Input: part model. Units: mm. Frame: model coordinates. Coordinates: 2 decimals unless noted, no trailing zeros. Loops run counter-clockwise (first coordinate to the right, second up) from the corner with the lowest first, then second, coordinate; pieces in that order, holes last. Notation, with made-up numbers: (-30, -33.5) -> (0, -33.5) arc R14 ccw to (0, -12.5) -> close; hole circle Ø10 at (5.25, 30.5). An arc over 180 degrees is marked (long way). Answer as a JSON object with one key per item and string values.
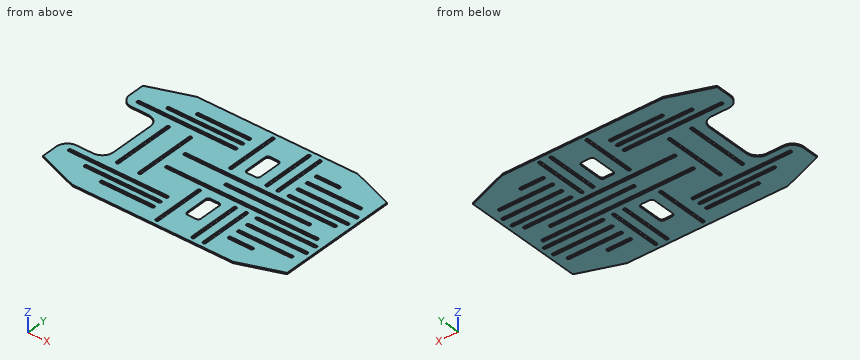
from build123d import *

# Parameters (mm, degrees)
BOSS_EXTRUDE1_DEPTH = 3.175
FILLET3_R           = 25.4
CUT_EXTRUDE3_DEPTH  = 4.175
SCALE1_SCALE        = 0.35


with BuildPart() as part:
    # Sketch1 → Boss-Extrude1 (new body)
    with BuildSketch(Plane.XY):
        Polygon((-279.4, 138.38935405), (-184.214073546, 173.034198), (184.214073546, 173.034198), (279.4, 138.38935405), (279.4, -138.38935405), (184.214073546, -173.034198), (-184.214073546, -173.034198), (-279.4, -138.38935405), (-279.4, -76.2), (-190.5, -76.2), (-190.5, 76.2), (-279.4, 76.2), align=None)
    extrude(amount=BOSS_EXTRUDE1_DEPTH)

    # Fillet3
    fillet3_edges = [part.edges().sort_by_distance(p)[0] for p in [
        (-279.4, -76.2, 1.5875),
        (-190.5, -76.2, 1.5875),
        (-190.5, 76.2, 1.5875),
        (-279.4, 76.2, 1.5875),
    ]]
    fillet(fillet3_edges, radius=FILLET3_R)

    # Sketch4 → Cut-Extrude3 (cut, through all)
    with BuildSketch(Plane.XY.offset(3.175)):
        with BuildLine():
            Line((-254, 98.6282), (-31.75, 98.6282))
            ThreePointArc((-31.75, 98.6282), (-28.3718, 95.25), (-31.75, 91.8718))
            Line((-31.75, 91.8718), (-254, 91.8718))
            ThreePointArc((-254, 91.8718), (-257.3782, 95.25), (-254, 98.6282))
        make_face()
        with BuildLine():
            Line((-201.660555159, 117.6782), (-31.75, 117.6782))
            ThreePointArc((-31.75, 117.6782), (-28.3718, 114.3), (-31.75, 110.9218))
            Line((-31.75, 110.9218), (-201.660555159, 110.9218))
            ThreePointArc((-201.660555159, 110.9218), (-205.038755159, 114.3), (-201.660555159, 117.6782))
        make_face()
        with BuildLine():
            Line((-149.321110319, 136.7282), (-31.75, 136.7282))
            ThreePointArc((-31.75, 136.7282), (-28.3718, 133.35), (-31.75, 129.9718))
            Line((-31.75, 129.9718), (-149.321110319, 129.9718))
            ThreePointArc((-149.321110319, 129.9718), (-152.699310319, 133.35), (-149.321110319, 136.7282))
        make_face()
        with BuildLine():
            Line((-161.7218, 69.85), (-161.7218, -69.85))
            ThreePointArc((-161.7218, -69.85), (-165.1, -73.2282), (-168.4782, -69.85))
            Line((-168.4782, -69.85), (-168.4782, 69.85))
            ThreePointArc((-168.4782, 69.85), (-165.1, 73.2282), (-161.7218, 69.85))
        make_face()
        with BuildLine():
            Line((-110.9218, 69.85), (-110.9218, -69.85))
            ThreePointArc((-110.9218, -69.85), (-114.3, -73.2282), (-117.6782, -69.85))
            Line((-117.6782, -69.85), (-117.6782, 69.85))
            ThreePointArc((-117.6782, 69.85), (-114.3, 73.2282), (-110.9218, 69.85))
        make_face()
        with BuildLine():
            Line((31.75, 114.3), (50.8, 114.3))
            ThreePointArc((50.8, 114.3), (55.290128061, 112.440128061), (57.15, 107.95))
            Line((57.15, 107.95), (57.15, 57.15))
            ThreePointArc((57.15, 57.15), (55.290128061, 52.659871939), (50.8, 50.8))
            Line((50.8, 50.8), (31.75, 50.8))
            ThreePointArc((31.75, 50.8), (27.259871939, 52.659871939), (25.4, 57.15))
            Line((25.4, 57.15), (25.4, 107.95))
            ThreePointArc((25.4, 107.95), (27.259871939, 112.440128061), (31.75, 114.3))
        make_face()
        with BuildLine():
            Line((3.3782, 160.334198), (3.3782, 44.45))
            ThreePointArc((3.3782, 44.45), (0, 41.0718), (-3.3782, 44.45))
            Line((-3.3782, 44.45), (-3.3782, 160.334198))
            ThreePointArc((-3.3782, 160.334198), (0, 163.712398), (3.3782, 160.334198))
        make_face()
        with BuildLine():
            Line((-88.9, 28.7782), (254, 28.7782))
            ThreePointArc((254, 28.7782), (257.3782, 25.4), (254, 22.0218))
            Line((254, 22.0218), (-88.9, 22.0218))
            ThreePointArc((-88.9, 22.0218), (-92.2782, 25.4), (-88.9, 28.7782))
        make_face()
        with BuildLine():
            Line((79.1718, 44.45), (79.1718, 160.334198))
            ThreePointArc((79.1718, 160.334198), (82.55, 163.712398), (85.9282, 160.334198))
            Line((85.9282, 160.334198), (85.9282, 44.45))
            ThreePointArc((85.9282, 44.45), (82.55, 41.0718), (79.1718, 44.45))
        make_face()
        with BuildLine():
            Line((111.3282, 160.334198), (111.3282, 44.45))
            ThreePointArc((111.3282, 44.45), (107.95, 41.0718), (104.5718, 44.45))
            Line((104.5718, 44.45), (104.5718, 160.334198))
            ThreePointArc((104.5718, 160.334198), (107.95, 163.712398), (111.3282, 160.334198))
        make_face()
        with BuildLine():
            Line((133.35, 124.0282), (184.214073546, 124.0282))
            ThreePointArc((184.214073546, 124.0282), (187.592273546, 120.65), (184.214073546, 117.2718))
            Line((184.214073546, 117.2718), (133.35, 117.2718))
            ThreePointArc((133.35, 117.2718), (129.9718, 120.65), (133.35, 124.0282))
        make_face()
        with BuildLine():
            Line((133.35, 98.6282), (254, 98.6282))
            ThreePointArc((254, 98.6282), (257.3782, 95.25), (254, 91.8718))
            Line((254, 91.8718), (133.35, 91.8718))
            ThreePointArc((133.35, 91.8718), (129.9718, 95.25), (133.35, 98.6282))
        make_face()
        with BuildLine():
            Line((133.35, 73.2282), (266.7, 73.2282))
            ThreePointArc((266.7, 73.2282), (270.0782, 69.85), (266.7, 66.4718))
            Line((266.7, 66.4718), (133.35, 66.4718))
            ThreePointArc((133.35, 66.4718), (129.9718, 69.85), (133.35, 73.2282))
        make_face()
        with BuildLine():
            Line((133.35, 47.8282), (266.7, 47.8282))
            ThreePointArc((266.7, 47.8282), (270.0782, 44.45), (266.7, 41.0718))
            Line((266.7, 41.0718), (133.35, 41.0718))
            ThreePointArc((133.35, 41.0718), (129.9718, 44.45), (133.35, 47.8282))
        make_face()
        with BuildLine():
            Line((-254, -98.6282), (-31.75, -98.6282))
            ThreePointArc((-31.75, -98.6282), (-28.3718, -95.25), (-31.75, -91.8718))
            Line((-31.75, -91.8718), (-254, -91.8718))
            ThreePointArc((-254, -91.8718), (-257.3782, -95.25), (-254, -98.6282))
        make_face()
        with BuildLine():
            Line((-201.660555159, -117.6782), (-31.75, -117.6782))
            ThreePointArc((-31.75, -117.6782), (-28.3718, -114.3), (-31.75, -110.9218))
            Line((-31.75, -110.9218), (-201.660555159, -110.9218))
            ThreePointArc((-201.660555159, -110.9218), (-205.038755159, -114.3), (-201.660555159, -117.6782))
        make_face()
        with BuildLine():
            Line((-149.321110319, -136.7282), (-31.75, -136.7282))
            ThreePointArc((-31.75, -136.7282), (-28.3718, -133.35), (-31.75, -129.9718))
            Line((-31.75, -129.9718), (-149.321110319, -129.9718))
            ThreePointArc((-149.321110319, -129.9718), (-152.699310319, -133.35), (-149.321110319, -136.7282))
        make_face()
        with BuildLine():
            Line((3.3782, -160.334198), (3.3782, -44.45))
            ThreePointArc((3.3782, -44.45), (0, -41.0718), (-3.3782, -44.45))
            Line((-3.3782, -44.45), (-3.3782, -160.334198))
            ThreePointArc((-3.3782, -160.334198), (0, -163.712398), (3.3782, -160.334198))
        make_face()
        with BuildLine():
            Line((-88.9, -28.7782), (254, -28.7782))
            ThreePointArc((254, -28.7782), (257.3782, -25.4), (254, -22.0218))
            Line((254, -22.0218), (-88.9, -22.0218))
            ThreePointArc((-88.9, -22.0218), (-92.2782, -25.4), (-88.9, -28.7782))
        make_face()
        with BuildLine():
            Line((79.1718, -44.45), (79.1718, -160.334198))
            ThreePointArc((79.1718, -160.334198), (82.55, -163.712398), (85.9282, -160.334198))
            Line((85.9282, -160.334198), (85.9282, -44.45))
            ThreePointArc((85.9282, -44.45), (82.55, -41.0718), (79.1718, -44.45))
        make_face()
        with BuildLine():
            Line((111.3282, -160.334198), (111.3282, -44.45))
            ThreePointArc((111.3282, -44.45), (107.95, -41.0718), (104.5718, -44.45))
            Line((104.5718, -44.45), (104.5718, -160.334198))
            ThreePointArc((104.5718, -160.334198), (107.95, -163.712398), (111.3282, -160.334198))
        make_face()
        with BuildLine():
            Line((133.35, -124.0282), (184.214073546, -124.0282))
            ThreePointArc((184.214073546, -124.0282), (187.592273546, -120.65), (184.214073546, -117.2718))
            Line((184.214073546, -117.2718), (133.35, -117.2718))
            ThreePointArc((133.35, -117.2718), (129.9718, -120.65), (133.35, -124.0282))
        make_face()
        with BuildLine():
            Line((133.35, -98.6282), (254, -98.6282))
            ThreePointArc((254, -98.6282), (257.3782, -95.25), (254, -91.8718))
            Line((254, -91.8718), (133.35, -91.8718))
            ThreePointArc((133.35, -91.8718), (129.9718, -95.25), (133.35, -98.6282))
        make_face()
        with BuildLine():
            Line((133.35, -73.2282), (266.7, -73.2282))
            ThreePointArc((266.7, -73.2282), (270.0782, -69.85), (266.7, -66.4718))
            Line((266.7, -66.4718), (133.35, -66.4718))
            ThreePointArc((133.35, -66.4718), (129.9718, -69.85), (133.35, -73.2282))
        make_face()
        with BuildLine():
            Line((133.35, -47.8282), (266.7, -47.8282))
            ThreePointArc((266.7, -47.8282), (270.0782, -44.45), (266.7, -41.0718))
            Line((266.7, -41.0718), (133.35, -41.0718))
            ThreePointArc((133.35, -41.0718), (129.9718, -44.45), (133.35, -47.8282))
        make_face()
        with BuildLine():
            Line((57.15, -107.95), (57.15, -57.15))
            ThreePointArc((57.15, -57.15), (55.290128061, -52.659871939), (50.8, -50.8))
            Line((50.8, -50.8), (31.75, -50.8))
            ThreePointArc((31.75, -50.8), (27.259871939, -52.659871939), (25.4, -57.15))
            Line((25.4, -57.15), (25.4, -107.95))
            ThreePointArc((25.4, -107.95), (27.259871939, -112.440128061), (31.75, -114.3))
            Line((31.75, -114.3), (50.8, -114.3))
            ThreePointArc((50.8, -114.3), (55.290128061, -112.440128061), (57.15, -107.95))
        make_face()
        with BuildLine():
            Line((25.4, 3.3782), (215.9, 3.3782))
            ThreePointArc((215.9, 3.3782), (219.2782, 0), (215.9, -3.3782))
            Line((215.9, -3.3782), (25.4, -3.3782))
            ThreePointArc((25.4, -3.3782), (22.0218, 0), (25.4, 3.3782))
        make_face()
    extrude(amount=-CUT_EXTRUDE3_DEPTH, mode=Mode.SUBTRACT)


with BuildPart() as part_1:
    # Scale1: scaled about (14.826143857, 0, 1.5875)
    add(part.part.scale(SCALE1_SCALE).moved(Location((9.636993507, 0, 1.031875))))


solid = part_1.part
1. Section query A-A (x = 44). Return loops of the section in (y, z), plus the area to 3 significant figures.
Reply:
{"outline": "(-60.56, 1.03) -> (-10.07, 1.03) -> (-10.07, 2.14) -> (-60.56, 2.14) -> close; (-7.71, 1.03) -> (-1.18, 1.03) -> (-1.18, 2.14) -> (-7.71, 2.14) -> close; (1.18, 1.03) -> (7.71, 1.03) -> (7.71, 2.14) -> (1.18, 2.14) -> close; (10.07, 1.03) -> (60.56, 1.03) -> (60.56, 2.14) -> (10.07, 2.14) -> close", "area": "127 mm2"}
2. Pin query (flat end, axial travel): P1, Ø0.6, axis at x = 86, z = 1.5, coming from the +Y side; P2, Ø0.6, axis at x = -69.5, z = 1.5, coming from the +Y side. Return the tip coordinate at first contact, or that it passes through.
Reply:
{"P1": "stops at y = 56.34", "P2": "stops at y = 55.33"}
3. Section query B-B (y = -51.5). Return loops of the section in (x, z).
Reply:
{"outline": "(-79.74, 1.03) -> (8.45, 1.03) -> (8.45, 2.14) -> (-79.74, 2.14) -> close; (10.82, 1.03) -> (37.35, 1.03) -> (37.35, 2.14) -> (10.82, 2.14) -> close; (39.71, 1.03) -> (46.24, 1.03) -> (46.24, 2.14) -> (39.71, 2.14) -> close; (48.6, 1.03) -> (99.01, 1.03) -> (99.01, 2.14) -> (48.6, 2.14) -> close"}
4. Line query: line 1 along X through (y, z) = (44.5, 1.7); line 2 along Y through (x, z) = (-50.5, 1.3); line 3 along Y through (x, z) = (3.5, 2.1). Output: solid intervals per line, ascending.
Reply:
{"line 1": "x = -88.15 to 8.45, 10.82 to 37.35, 39.71 to 46.24, 48.6 to 107.43", "line 2": "y = -60.56 to -41.19, -38.82 to -34.52, -32.16 to 32.16, 34.52 to 38.82, 41.19 to 60.56", "line 3": "y = -60.56 to -10.07, -7.71 to 7.71, 10.07 to 60.56"}
5. Section query C-C (z = 1.3). Count the separate pieces of the cut face and the enclosed holes in it, plus the area to 3 significant figures.
Reply:
{"separate pieces": "1", "enclosed holes": "27", "area": "17,500 mm2"}
